Read the model definition and answer for the solid it produces. Units are mm, in the model's axes. A direction names the side the tool comes from. Round coordinates to 2 decimals unless told otherwise and drop trailing zeros. Order: outer loops, then holes, each group sorted by start corner. A loop starts at its lowest first (then second) coordinate and runs counter-clockwise, first axis right, second up. Notation, with made-up numbers: (41.5, 84) -> (49.5, 84) arc R28 cw to (49.5, 107) -> close; hole circle Ø10 at (-21, 66). An arc over 180 degrees is marked (long way). Use a Markdown table: item, result. Add a question column.
1. Section A-A, the plane y = -0.75 is taken. Give the vertices of the cut face in (x, z).
2. Section C-C, the plane x = -6.25 is taken. Give the vertices of the cut face in (y, z), then the cut area to 3 significant figures.
3. Section D-D, the plane y = -5.75 is taken. Give the vertices of the cut face in (x, z).
4. Given pin 1 (2 mm diameter, centred on y = -5, z = -11.5, fed in from +X); pin 2 (6 mm diameter, centred on x = -3, z = -17, fed in from +Y); pin 3 (6 mm diameter, centred on x = 2.5, z = -8, fed in from -Y), each flat-ended and moving along its own axis, determine where each tip first touches the part or whether it passes through.
5. For faces 1 (the face through (-6.03, -4.79, 2.5)), 2 (the face through (-3.13, -3.53, -15.65)), determine the directions among +Z, -Z, +X, -X, +Y, -Y from which every point of the face is accessible in a straight line to the end or side of a thin tool.
6. Consider L1, parallel to Z at x = -2.75, y = -4; L2, parallel to X at y = -1.75, z = -16.5; L3, parallel to X at y = -3.75, z = -24. Determine where each line is inside the solid, lowest interval first. Write a range as [from, to].
Autodesk Inventor part; units mm, degrees
ref_plane "YZ Plane" through (0, 0, 0) normal (1, 0, 0) x (0, 1, 0)
ref_plane "XZ Plane" through (0, 0, 0) normal (0, 1, 0) x (-1, 0, 0)
ref_plane "XY Plane" through (0, 0, 0) normal (0, 0, 1) x (1, 0, 0)
sketch "Sketch1" plane through (0, 0, 0) normal (0, 0, 1) x (1, 0, 0)
  circle A0 centre (-0.6115, -1.5992) radius 3.175
  line L0 (-7.8705, -1.5992) -> (-4.241, 4.6873)
  line L1 (-4.241, 4.6873) -> (3.018, 4.6873)
  line L2 (3.018, 4.6873) -> (6.6475, -1.5992)
  line L3 (6.6475, -1.5992) -> (3.018, -7.8857)
  line L4 (3.018, -7.8857) -> (-4.241, -7.8857)
  line L5 (-4.241, -7.8857) -> (-7.8705, -1.5992)
  dimension "d10" = 12.573
extrude "Extrusion1" add sketch "Sketch1" against normal blind 31.75 contours A0
extrude "Extrusion2" add sketch "Sketch1" along normal blind 5.08 contours A0 | L0 L1 L2 L3 L4 L5
thread "Thread1"
properties part number "HW-00037"
Verdict:
| question | item | result |
|---|---|---|
| 1 | outline | (-7.38, 0) -> (-3.67, 0) -> (-3.67, -31.75) -> (2.45, -31.75) -> (2.45, 0) -> (6.16, 0) -> (6.16, 5.08) -> (-7.38, 5.08) -> close |
| 2 | outline | (-4.41, 0) -> (1.21, 0) -> (1.21, 5.08) -> (-4.41, 5.08) -> close |
| 2 | area | 28.5 mm2 |
| 3 | outline | (-5.47, 0) -> (4.25, 0) -> (4.25, 5.08) -> (-5.47, 5.08) -> close |
| 4 | pin 1 | stops at x = 1.47 |
| 4 | pin 2 | stops at y = 1.58 |
| 4 | pin 3 | stops at y = -4.77 |
| 5 | face 1 | +Z, -Z, -X, -Y |
| 5 | face 2 | -Z |
| 6 | L1 | z = [0, 5.08] |
| 6 | L2 | x = [-3.78, 2.56] |
| 6 | L3 | x = [-2.95, 1.72] |
